from build123d import *

# Parameters (mm, degrees)
F0_R     = 75
F1_DEPTH = 60
F3_W     = 7.8857280314
F3_H     = 170.0287312269
F5_ANGLE = 30
F7_R     = 5
F8_R     = 5


with BuildPart() as f1:
    # F0 (on Front) → F1 (new body)
    with BuildSketch(Plane.XZ):
        Circle(F0_R)
    extrude(amount=F1_DEPTH)

    # F3 (on face) → F4 (revolve)
    with BuildSketch(Plane.XZ.offset(60)):
        Polygon((0, 90.5750542879), (0, 82.0537060499), (7.8857280314, 82.0537060499), (29.3278116733, 82.0537060499), (29.3278116733, 90.5750542879), align=None)
        with Locations((3.9428640157, -2.9606595635)):
            Rectangle(F3_W, F3_H)
    revolve(axis=Axis((0, -60, -2.9606595635), (0, 0, -1)))


with BuildPart() as f1_1:
    # F5: moved
    add(f1.part.rotate(Axis((0, 0, 0), (0, -1, 0)), F5_ANGLE))

    # F6: F1 across plane


with BuildPart() as f1_2:
    add(f1_1.part)
    add(f1_1.part.mirror(Plane.YZ))

    # F7
    f7_edges = [f1_2.edges().sort_by_distance(p)[0] for p in [
        (-70.686157, -60, 63.776392),
    ]]
    fillet(f7_edges, radius=F7_R)

    # F8
    f8_edges = [f1_2.edges().sort_by_distance(p)[0] for p in [
        (70.686157, -60, 63.776392),
    ]]
    fillet(f8_edges, radius=F8_R)


solid = f1_2.part
Source: CAD feature listing. Evaluate the final solid. Frame: model axes, mm. A direction names the side the tool comes from. Give positions to 0.01 mm unless a question says otherwise; leave off trailing zeros. Order: outer loops, then holes, each group sorted by start corner. A loop starts at its lowest first (then second) coordinate and runs counter-clockwise, first axis right, second up. Notation, with made-up numbers: (31, 36.5) -> (78, 36.5) arc R12 cw to (78, 50.5) -> close; hole circle Ø1 at (68.5, 48). An arc over 180 degrees is marked (long way). Use a Markdown table: item, result.
1) Mould query, pull axis Z, two halves, no side actions, for faces 1 (the flat face through (-1, 0, 0)), 2 (the flat face through (-45.58, -60.34, 78.27)), 3 (the flat face through (46, -60, 2)). Classes: +Z half, -Z half, draft (parallel to the pull), parting line (faces both ways), or undercut.
Answer list:
| item | result |
|---|---|
| face 1 | draft |
| face 2 | +Z half |
| face 3 | undercut |
2) Section query A-A, the plane y = -24.5. Return the cut outline in (x, z).
Answer list:
| item | result |
|---|---|
| outline | circle Ø150 at (0, 0) |
3) Contact query for flat-ended pins moving along their axis: P1, Ø20, axis at x = -35, z = 22.5, coming from the -Y side; P2, Ø18, axis at x = -10, z = 48, coming from the -Y side; P3, Ø6, axis at x = -24, y = -28.5, coming from the -Z side. Output: stop coordinate, or through.
Answer list:
| item | result |
|---|---|
| P1 | y = -60 |
| P2 | y = -64.69 |
| P3 | z = -72 |
4) Ray query, line 1 along Y through (x, z) = (-24.5, 67); line 2 along Z through (x, y) = (-37, -34); line 3 along X through (y, z) = (-8.5, 35). Return the intervals inside material, ascending. Write a range as [from, to].
Answer list:
| item | result |
|---|---|
| line 1 | [-60, 0] |
| line 2 | [-65.24, 65.24], [73.39, 81.93] |
| line 3 | [-66.33, 66.33] |
5) Reachability of faces 4 (the flat face through (-3, -60, -52)), 5 (the flat face through (-46.315, -53.893, 68.007)), 6 (the flat face through (2, -60, 53)), 7 (the flat face through (-44.083, -60.11, -76.133)) from +Z, -Z, +X, -X, +Y, -Y: full face, straight path, thin tool, end or side. Return the list, or none.
Answer list:
| item | result |
|---|---|
| face 4 | -Z, -Y |
| face 5 | none |
| face 6 | -Y |
| face 7 | -Z, -X, +Y, -Y |
